Could you check a few things on this model? Use its own coordinates, in mm. A direction names the side the tool comes from. Coordinates: 2 decimals unless noted, no trailing zeros. Write each loop counter-clockwise with the first axis right and the second up, starting at its lowest first coordinate (ties: lowest second). Pieces come first, ordered by that corner, then holes.
```python
from build123d import *

# Parameters (mm, degrees)
F1_DEPTH = 3
F2_W     = 6.6697
F2_H     = 2.858443
F2_R     = 1.413331
F3_DEPTH = 25


with BuildPart() as f1:
    # F0 (on Top) → F1 (new body)
    with BuildSketch(Plane.XY):
        Polygon((7.5, 11.661676), (-47.5, 11.661676), (-47.5, -11.661676), (-47.5, -23.794964), (-35.409175, -23.794964), (-35.409175, -11.661676), (-19.262591, -11.661676), (-19.262591, -15.296764), (-14.446942, -15.296764), (-14.446942, -11.661676), (7.5, -11.661676), (7.5, -4.661676), (11.5, -4.661676), (11.5, -11.661676), (44.5, -11.661676), (44.5, -14.661676), (47.5, -14.661676), (47.5, -11.661676), (47.5, 11.661676), (11.5, 11.661676), (11.5, 4.661676), (7.5, 4.661676), align=None)
    extrude(amount=F1_DEPTH)

    # F2 (on face) → F3 (cut)
    with BuildSketch(Plane(origin=(0, 0, 0), x_dir=(1, 0, 0), z_dir=(0, 0, -1))):
        with Locations((-41.646808, 19.972993)):
            Rectangle(F2_W, F2_H)
        with Locations((9.805162, 0)):
            Circle(F2_R)
    extrude(amount=-F3_DEPTH, mode=Mode.SUBTRACT)


solid = f1.part
```
1. For pin 1 (12 mm diameter, centred on x = -17, y = -0.5, fed in from -Z); pin 2 (1.5 mm diameter, centred on x = 8.5, z = 1.5, fed in from +Y); pin 3 (1.5 mm diameter, centred on y = -15.5, z = 2, fed in from +X), each with a flat end and sliding along its axis, tell me the tip position at first contact or that it passes through.
Verdict:
pin 1: stops at z = 0
pin 2: stops at y = 4.66
pin 3: stops at x = -14.45
2. I want a section at B-B on z = 1.6. Please give me the cut outline in (x, y).
Verdict:
outline: (-47.5, -23.79) - (-35.41, -23.79) - (-35.41, -11.66) - (-19.26, -11.66) - (-19.26, -15.3) - (-14.45, -15.3) - (-14.45, -11.66) - (7.5, -11.66) - (7.5, -4.66) - (11.5, -4.66) - (11.5, -11.66) - (44.5, -11.66) - (44.5, -14.66) - (47.5, -14.66) - (47.5, 11.66) - (11.5, 11.66) - (11.5, 4.66) - (7.5, 4.66) - (7.5, 11.66) - (-47.5, 11.66) - close; hole (-44.98, -21.4) - (-38.31, -21.4) - (-38.31, -18.54) - (-44.98, -18.54) - close; hole circle Ø2.83 at (9.81, 0)
3. I want a section at D-D on x = 14.5. Please give me the cut outline in (y, z).
Verdict:
outline: (-11.66, 0) - (11.66, 0) - (11.66, 3) - (-11.66, 3) - close
4. If we mould it in two halves opening along X, with no side actions, what happens to faces 1 (the face through (44.5, -13, 1)), 2 (the face through (-1, -2, 0)), 3 (the face through (47.5, -2, 1))? For each: pulls with the +X half, pulls with the -X half, needs draft (parallel to the pull), parting line crosses it, or undercut.
Verdict:
face 1: undercut
face 2: needs draft
face 3: pulls with the +X half
5. I want a section at C-C on y = -5.5. Please give me the cut outline in (x, z), plus the area to 3 significant figures.
Verdict:
outline: (-47.5, 0) - (7.5, 0) - (7.5, 3) - (-47.5, 3) - close; (11.5, 0) - (47.5, 0) - (47.5, 3) - (11.5, 3) - close
area: 273 mm2
6. I want a section at A-A on y = 0. Please give me the cut outline in (x, z), plus the area to 3 significant figures.
Verdict:
outline: (-47.5, 0) - (8.39, 0) - (8.39, 3) - (-47.5, 3) - close; (11.22, 0) - (47.5, 0) - (47.5, 3) - (11.22, 3) - close
area: 277 mm2
7. On a 3-axis mill with a long thin cutter (end or side, diameter ignored), from which of +Z, -Z, +X, -X, +Y, -Y can I reach the whole of each face in a straight line? I mean faces 4 (the face through (7.5, 8, 1)), 5 (the face through (-38.312, -20, 1)), 6 (the face through (7.5, -8, 1)). Say none if no direction works.
Verdict:
face 4: +Z, -Z, +Y
face 5: +Z, -Z
face 6: +Z, -Z, -Y
8. Please list where these lines run through material, in increasing order: line 1 along X through (y, z) = (8.5, 1.1); line 2 along X through (y, z) = (-14, 2.45); line 3 along X through (y, z) = (-21, 1.25).
Verdict:
line 1: x = -47.5 to 7.5, 11.5 to 47.5
line 2: x = -47.5 to -35.41, -19.26 to -14.45, 44.5 to 47.5
line 3: x = -47.5 to -44.98, -38.31 to -35.41
